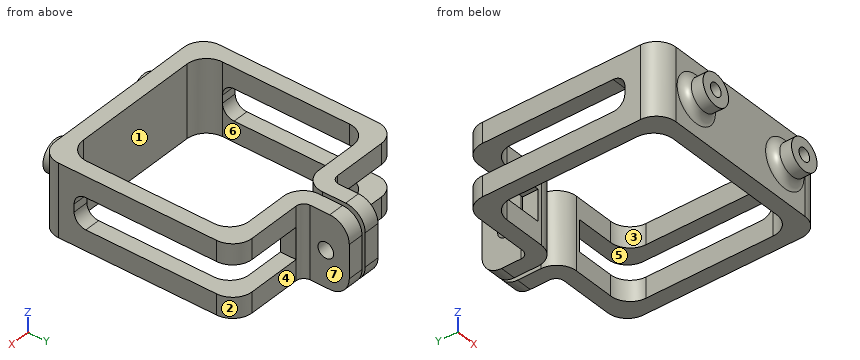
from build123d import *
from OCP.BRepFilletAPI import BRepFilletAPI_MakeFillet

# Parameters (mm, degrees)
SKETCH1_W                    = 50.5
SKETCH1_H                    = 50.5
SKETCH1_W_2                  = 42.5
SKETCH1_H_2                  = 42.5
BOSS_EXTRUDE1_DEPTH          = 9.25
SKETCH2_W                    = 1
SKETCH2_H                    = 4
CUT_EXTRUDE1_DEPTH           = 41.21660105
SKETCH3_W                    = 4
SKETCH3_H                    = 12
BOSS_EXTRUDE2_DEPTH          = 18.5
SKETCH4_R                    = 2
CUT_EXTRUDE2_DEPTH           = 49.561172762
FILLET1_R1                   = 5
FILLET1_R2                   = 2
SKETCH5_W                    = 18.75
SKETCH5_H                    = 8
CUT_EXTRUDE3_DEPTH           = 41.5
FILLET2_R                    = 3
SKETCH6_R                    = 4
BOSS_EXTRUDE3_DEPTH          = 5
SKETCH7_R                    = 1.675
CUT_EXTRUDE4_DEPTH           = 5
CUT_EXTRUDE4_DRAFT           = -2
CUT_EXTRUDE4_PROFILE_2_DEPTH = 5
CUT_EXTRUDE4_PROFILE_2_DRAFT = -2
FILLET3_R                    = 2


with BuildPart() as part:
    # Sketch1 → Boss-Extrude1 (new, symmetric)
    with BuildSketch(Plane.XY):
        Rectangle(SKETCH1_W, SKETCH1_H)
        Rectangle(SKETCH1_W_2, SKETCH1_H_2, mode=Mode.SUBTRACT)
    extrude(amount=BOSS_EXTRUDE1_DEPTH, both=True)

    # Sketch2 → Cut-Extrude1 (cut, through all)
    with BuildSketch(Plane.XY.offset(9.25)):
        with Locations((0, 23.25)):
            Rectangle(SKETCH2_W, SKETCH2_H)
    extrude(amount=-CUT_EXTRUDE1_DEPTH, mode=Mode.SUBTRACT)

    # Sketch3 → Boss-Extrude2 (add)
    with BuildSketch(Plane.XY.offset(9.25)):
        with Locations((2.5, 31.25)):
            Rectangle(SKETCH3_W, SKETCH3_H)
        with Locations((-2.5, 31.25)):
            Rectangle(SKETCH3_W, SKETCH3_H)
    extrude(amount=-BOSS_EXTRUDE2_DEPTH)

    # Sketch4 → Cut-Extrude2 (cut, through all)
    with BuildSketch(Plane(origin=(4.5, 0, 0), x_dir=(0, 0, -1), z_dir=(1, 0, 0))):
        with Locations((0, 31.25)):
            Circle(SKETCH4_R)
    extrude(amount=-CUT_EXTRUDE2_DEPTH, mode=Mode.SUBTRACT)

    # Fillet1: one fillet with a radius per group of edges: ONE call of the kernel's fillet builder (fillet() takes one radius for all edges)
    fillet1_edges_1 = [part.edges().sort_by_distance(p)[0] for p in [
        (-21.25, 21.25, 0),
        (-21.25, -21.25, 0),
        (21.25, -21.25, 0),
        (21.25, 21.25, 0),
        (-0.5, 21.25, 0),
        (0.5, 21.25, 0),
        (2.5, 37.25, 9.25),
        (2.5, 37.25, -9.25),
        (-2.5, 37.25, 9.25),
        (-2.5, 37.25, -9.25),
        (25.25, -25.25, 0),
        (-25.25, -25.25, 0),
        (-25.25, 25.25, 0),
        (25.25, 25.25, 0),
    ]]
    fillet1_edges_2 = [part.edges().sort_by_distance(p)[0] for p in [
        (4.5, 25.25, 0),
        (-4.5, 25.25, 0),
    ]]
    fillet1 = BRepFilletAPI_MakeFillet(part.part.solid().wrapped)
    for e in fillet1_edges_1:
        fillet1.Add(FILLET1_R1, e.wrapped)
    for e in fillet1_edges_2:
        fillet1.Add(FILLET1_R2, e.wrapped)
    add(Compound.cast(fillet1.Shape()), mode=Mode.REPLACE)

    # Sketch5 → Cut-Extrude3 (cut)
    with BuildSketch(Plane(origin=(0, 25.25, 0), x_dir=(1, 0, 0), z_dir=(0, 1, 0))):
        with Locations((-15.875, 0)):
            Rectangle(SKETCH5_W, SKETCH5_H)
        with Locations((15.875, 0)):
            Rectangle(SKETCH5_W, SKETCH5_H)
    extrude(amount=-CUT_EXTRUDE3_DEPTH, mode=Mode.SUBTRACT)

    # Fillet2
    fillet2_edges = [part.edges().sort_by_distance(p)[0] for p in [
        (-23.25, -16.25, 4),
        (-23.25, -16.25, -4),
        (23.25, -16.25, -4),
        (23.25, -16.25, 4),
    ]]
    fillet(fillet2_edges, radius=FILLET2_R)

    # Sketch6 → Boss-Extrude3 (add)
    with BuildSketch(Plane(origin=(0, -25.25, 0), x_dir=(-1, 0, 0), z_dir=(0, -1, 0))):
        with Locations((-13.875, 0)):
            Circle(SKETCH6_R)
        with Locations((13.875, 0)):
            Circle(SKETCH6_R)
    extrude(amount=BOSS_EXTRUDE3_DEPTH)


with BuildPart() as cut_extrude4_tool:
    # Sketch7 → Cut-Extrude4 (with draft: the straight prism first)
    with BuildSketch(Plane(origin=(0, -30.25, 0), x_dir=(-1, 0, 0), z_dir=(0, -1, 0))):
        with Locations((-13.875, 0)):
            Circle(SKETCH7_R)
    extrude(amount=-CUT_EXTRUDE4_DEPTH)
    # Cut-Extrude4: the draft: its side faces are tilted about the plane it starts from
    cut_extrude4_sides = [cut_extrude4_tool.faces().sort_by_distance(p)[0] for p in [
        (15.55, -27.75, 0),
    ]]
    draft(cut_extrude4_sides, Plane(origin=(0, -30.25, 0), x_dir=(-1, 0, 0), z_dir=(0, -1, 0)), CUT_EXTRUDE4_DRAFT)


with BuildPart() as part_1:
    add(part.part)

    # Cut-Extrude4: cut by cut_extrude4_tool
    add(cut_extrude4_tool.part, mode=Mode.SUBTRACT)


with BuildPart() as cut_extrude4_profile_2_tool:
    # Sketch7 → Cut-Extrude4 profile 2 (with draft: the straight prism first)
    with BuildSketch(Plane(origin=(0, -30.25, 0), x_dir=(-1, 0, 0), z_dir=(0, -1, 0))):
        with Locations((13.875, 0)):
            Circle(SKETCH7_R)
    extrude(amount=-CUT_EXTRUDE4_PROFILE_2_DEPTH)
    # Cut-Extrude4 profile 2: the draft: its side faces are tilted about the plane it starts from
    cut_extrude4_profile_2_sides = [cut_extrude4_profile_2_tool.faces().sort_by_distance(p)[0] for p in [
        (-12.2, -27.75, 0),
    ]]
    draft(cut_extrude4_profile_2_sides, Plane(origin=(0, -30.25, 0), x_dir=(-1, 0, 0), z_dir=(0, -1, 0)), CUT_EXTRUDE4_PROFILE_2_DRAFT)


with BuildPart() as part_2:
    add(part_1.part)

    # Cut-Extrude4 profile 2: cut by cut_extrude4_profile_2_tool
    add(cut_extrude4_profile_2_tool.part, mode=Mode.SUBTRACT)

    # Fillet3
    fillet3_edges = [part_2.edges().sort_by_distance(p)[0] for p in [
        (17.875, -25.25, 0),
        (-9.875, -25.25, 0),
    ]]
    fillet(fillet3_edges, radius=FILLET3_R)


solid = part_2.part
Verification items for the finished model (mm, model axes). Face numbers are marked on the shaded views. A direction names the side the tool comes from. Give positions to 0.01 mm unless a question says otherwise; leave off trailing zeros. Loops run counter-clockwise (first coordinate to the right, second up) from the corner with the lowest first, then second, coordinate; pieces in that order, holes last.
1. Material ranges on probe 1 along Y at (x, z) = (12, 8.75); probe 2 along Z at (x, y) = (-3, 31); probe 3 along Y at (x, z) = (-1.45, 0), recorded low to high.
Derived:
probe 1: y = -25.25 to -21.25, 21.25 to 25.25
probe 2: z = -9.25 to -1.98, 1.98 to 9.25
probe 3: y = -25.25 to -21.25, 23.32 to 29.25, 33.25 to 37.25
2. Tool access check on the marked faces 5, 6 and 7. Record the directions out of +Z, -Z, +X, -X, +Y, -Y that give a thin tool (end or side, any length) a straight path to the whole face; none if there is none.
Derived:
face 5: +X, +Y
face 6: +Z, -Z
face 7: +Z, -Z, +X, +Y
3. Cross-section at D-D on y = 10.5. Record the cut outline in (x, z).
Derived:
outline: (-25.25, -9.25) - (-21.25, -9.25) - (-21.25, -4) - (-25.25, -4) - close; (-25.25, 4) - (-21.25, 4) - (-21.25, 9.25) - (-25.25, 9.25) - close; (21.25, -9.25) - (25.25, -9.25) - (25.25, -4) - (21.25, -4) - close; (21.25, 4) - (25.25, 4) - (25.25, 9.25) - (21.25, 9.25) - close
4. Go/stop test with flat-tipped pins: P1, Ø1, axis at x = 15, z = 5, coming from the -Y side; P2, Ø4, axis at x = -18.5, y = 7, coming from the +Z side; P3, Ø3, axis at y = 33, z = -2.5, coming from the -X side; P4, Ø3, axis at y = 23.5, z = -2, coming from the -X side. Record where each tip stops, or that it passes through.
Derived:
P1: stops at y = -25.8
P2: passes through
P3: stops at x = -4.5
P4: stops at x = -6.5
5. Release check for a two-part mould opening along X. For the marked faces 1, 2, 3 and 4 record: +X half, -X half, draft (parallel to the pull), parting line (faces both ways), or undercut.
Derived:
face 1: undercut
face 2: +X half
face 3: undercut
face 4: draft
6. Cross-section at B-B on x = 2. Record the cut outline in (y, z), and give its area (3 significant figures).
Derived:
outline: (-25.25, -9.25) - (-21.25, -9.25) - (-21.25, 9.25) - (-25.25, 9.25) - close; (22.68, -9.25) - (32.25, -9.25) arc R5 ccw to (37.25, -4.25) - (37.25, 4.25) arc R5 ccw to (32.25, 9.25) - (22.68, 9.25) - close; hole circle Ø4 at (31.25, 0)
area: 320 mm2
7. Cross-section at C-C on z = 0. Count the separate pieces of the cut face and the enclosed holes in it, and give its area (3 significant figures).
Derived:
separate pieces: 5
enclosed holes: 0
area: 397 mm2
8. Cross-section at A-A on y = 31.25. Record the cut outline in (x, z), and give its area (3 significant figures).
Derived:
outline: (-4.5, -9.25) - (-0.5, -9.25) - (-0.5, -2) - (-4.5, -2) - close; (-4.5, 2) - (-0.5, 2) - (-0.5, 9.25) - (-4.5, 9.25) - close; (0.5, -9.25) - (4.5, -9.25) - (4.5, -2) - (0.5, -2) - close; (0.5, 2) - (4.5, 2) - (4.5, 9.25) - (0.5, 9.25) - close
area: 116 mm2
